Check sheet for the modelled part. Datum: model origin and axes. Units: mm. A direction names the side the tool comes from. Give positions to 0.01 mm unless a question says otherwise; leave off trailing zeros. Loops run counter-clockwise (first coordinate to the right, second up) from the corner with the lowest first, then second, coordinate; pieces in that order, holes last. Notation, with made-up numbers: (42.25, -12.5) - (86.25, -12.5) arc R12 ccw to (86.25, -0.5) - close; hole circle Ø6 at (-19.5, 49.5). An arc over 180 degrees is marked (long way). Answer in a Markdown table with one row per item. Add a question column.
(1) Draft check along Y on faces 1 (the face through (-4, 1, 0)), 2 (the face through (-2.96, -3.3, 10.45)), 3 (the face through (-5.22, 9.63, 7.31)), 4 (the face through (-3, -6.868, 6)). Enter one of: released by +Y, released by -Y, zero draft, split by the parting line, or undercut.
(2) Sectioned sample at D-D on z = 11.25. Enter the section's corners in (x, y), then the cut area to 3 significant figures.
(3) Sectioned sample at B-B on y = 9.5. Enter the section's corners in (x, z).
(4) Sectioned sample at A-A on z = 6. Enter the section's corners in (x, y).
(5) Set-up check for faces 5 (the face through (-7, 8.132, 6)), 6 (the face through (-2, -0.868, 6)), 7 (the face through (-7.5, 9, 5)): record each of +Z, -Z, +X, -X, +Y, -Y from which the full face is reachable in a straight line by a thin tool's end or side.
(6) Thickness scan on L1, parallel to Z at x = -5.75, y = 10.5; L2, parallel to Y at x = -3.6, z = 9; L3, parallel to Y at x = -6.05, z = 6. Record the ranges inside material, lowest first.
(7) Go/stop test with flat-tipped pins: P1, Ø4, axis at x = -3, y = 2, coming from the -Z side; P2, Ø1.7, axis at y = -3.37, z = 3, coming from the -X side; P3, Ø3.5, axis at y = 3, z = 8.5, coming from the -X side; P4, Ø6, axis at y = 5.5, z = 7, coming from the +X side. Record where each tip stops, or that it passes through.
(8) Sectioned sample at C-C on x = -6.5. Enter the section's corners in (y, z), then the cut area to 3 significant figures.
from build123d import *

# Parameters (mm, degrees)
BOSS_EXTRUDE1_DEPTH         = 12
M2_5_CLEARANCE_HOLE1_D      = 2.9
TAP_DRILL_FOR_M4X0_7_TAP1_D = 3.3


with BuildPart() as part:
    # Sketch1 → Boss-Extrude1 (new body)
    with BuildSketch(Plane.XY):
        Polygon((0, -6.868421053), (-6, -6.868421053), (-6, 8.131578947), (-7.5, 8.131578947), (-7.5, 13.131578947), (-3, 13.131578947), (-3, -0.868421053), (0, -0.868421053), align=None)
    extrude(amount=BOSS_EXTRUDE1_DEPTH)

    # M2.5 Clearance Hole1 (through all)
    with Locations(Plane.ZY.offset(6)):
        with Locations((3, -3.368421053), (9, -3.368421053)):
            Hole(M2_5_CLEARANCE_HOLE1_D / 2)

    # Tap Drill for M4x0.7 Tap1 (through all)
    with Locations(Plane.ZY.offset(7.5)):
        with Locations((6, 10.631578947)):
            Hole(TAP_DRILL_FOR_M4X0_7_TAP1_D / 2)


solid = part.part
Reply:
| question | item | result |
|---|---|---|
| 1 | face 1 | zero draft |
| 1 | face 2 | undercut |
| 1 | face 3 | undercut |
| 1 | face 4 | released by -Y |
| 2 | outline | (-7.5, 8.13) - (-6, 8.13) - (-6, -6.87) - (0, -6.87) - (0, -0.87) - (-3, -0.87) - (-3, 13.13) - (-7.5, 13.13) - close |
| 2 | area | 85.5 mm^2 |
| 3 | outline | (-7.5, 0) - (-3, 0) - (-3, 4.8) - (-7.5, 4.8) - close; (-7.5, 7.2) - (-3, 7.2) - (-3, 12) - (-7.5, 12) - close |
| 4 | outline | (-7.5, 8.13) - (-6, 8.13) - (-6, -6.87) - (0, -6.87) - (0, -0.87) - (-3, -0.87) - (-3, 8.98) - (-7.5, 8.98) - close; (-7.5, 12.28) - (-3, 12.28) - (-3, 13.13) - (-7.5, 13.13) - close |
| 5 | face 5 | +Z, -Z, -X, -Y |
| 5 | face 6 | +Z, -Z, +X, +Y |
| 5 | face 7 | +Z, -Z, -X, +Y, -Y |
| 6 | L1 | 0 to 4.36, 7.64 to 12 |
| 6 | L2 | -6.87 to -4.82, -1.92 to 13.13 |
| 6 | L3 | 8.13 to 8.98, 12.28 to 13.13 |
| 7 | P1 | z = 0 |
| 7 | P2 | through |
| 7 | P3 | x = -6 |
| 7 | P4 | x = -3 |
| 8 | outline | (8.13, 0) - (13.13, 0) - (13.13, 12) - (8.13, 12) - close; hole circle Ø3.3 at (10.63, 6) |
| 8 | area | 51.4 mm^2 |
